For this review, use the dimensioned drawing (mm, ordinates from the lowest corner) and the shaded views. A direction names the side the tool comes from. Round coordinates to 2 decimals unless told otherwise and drop trailing zeros. Write each loop counter-clockwise with the first axis right and the second up, starting at its lowest first coordinate (ties: lowest second). Pieces come first, ordered by that corner, then holes. Notation, with made-up numbers: M -13.75,-15 L -2.75,-15 A13 ccw -2.75,-7 Z; hole C -20,66.5 d8. An arc over 180 degrees is marked long. Answer in a Markdown table with one row per item.
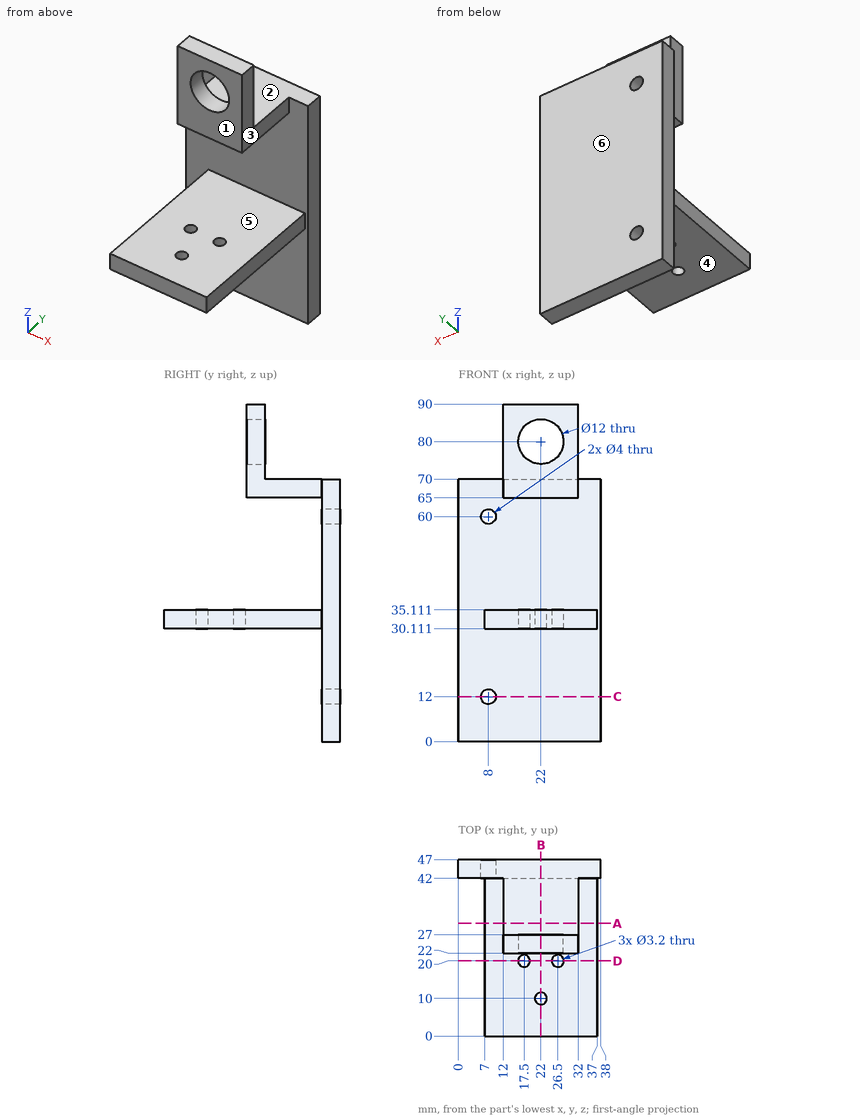
Q1. Take a section at A-A (y = 30). State the section outline as (x, z) points, then the cut area to 3 significant figures.
Found:
| item | result |
|---|---|
| outline | M 7,30.11 L 37,30.11 L 37,35.11 L 7,35.11 Z; M 12,65 L 32,65 L 32,70 L 12,70 Z |
| area | 250 mm² |
Q2. Machinability: for the marked faces 1, 2 and 3, which of the approach directions +Z, -Z, +X, -X, +Y, -Y give a long, thin tool a straight path to every point of the face, cutting with its end or side? Answer none if there is none.
Found:
| item | result |
|---|---|
| face 1 | +Z, +X, -X, -Y |
| face 2 | +Z, +X, -X, +Y |
| face 3 | +Z, +X, -Y |
Q3. For probe 1 along Z at (x, y) = (21.5, 22.5); probe 2 along Z at (x, y) = (26, 34.5); probe 3 along Y at (x, z) = (36.5, 56), list the stretches that pass through material, from the lowest coordinate up.
Found:
| item | result |
|---|---|
| probe 1 | 30.11 to 35.11, 65 to 74.02, 85.98 to 90 |
| probe 2 | 30.11 to 35.11, 65 to 70 |
| probe 3 | 42 to 47 |
Q4. Mouldability with a two-part tool opening along Z and no side actions: class the marked faces 4, 5 and 6 as +Z half, -Z half, draft (parallel to the pull), parting line (faces both ways), or undercut.
Found:
| item | result |
|---|---|
| face 4 | -Z half |
| face 5 | undercut |
| face 6 | draft |
Q5. Insertion check: P1, Ø10, axis at x = 10, y = 38, coming from the +Z side; P2, Ø12, axis at x = 15.5, y = 35, coming from the -Z side; P3, Ø14, axis at x = 22, z = 80, coming from the +Y side. Each pin has a flat end and moves straight along its axis. Give the tip position at first contact, or say it passes through.
Found:
| item | result |
|---|---|
| P1 | z = 70 |
| P2 | z = 30.11 |
| P3 | y = 27 |
Q6. Take a section at D-D (y = 20). State the section outline as (x, z) points.
Found:
| item | result |
|---|---|
| outline | M 7,30.11 L 15.9,30.11 L 15.9,35.11 L 7,35.11 Z; M 19.1,30.11 L 24.9,30.11 L 24.9,35.11 L 19.1,35.11 Z; M 28.1,30.11 L 37,30.11 L 37,35.11 L 28.1,35.11 Z |
Q7. Take a section at B-B (x = 22). State the section outline as (y, z) points, then the cut area to 3 significant figures.
Found:
| item | result |
|---|---|
| outline | M 0,30.11 L 8.4,30.11 L 8.4,35.11 L 0,35.11 Z; M 11.6,30.11 L 42,30.11 L 42,0 L 47,0 L 47,70 L 27,70 L 27,74 L 22,74 L 22,65 L 42,65 L 42,35.11 L 11.6,35.11 Z; M 22,86 L 27,86 L 27,90 L 22,90 Z |
| area | 684 mm² |
Q8. Take a section at C-C (z = 12). State the section outline as (x, y) points, then the cut area to 3 significant figures.
Found:
| item | result |
|---|---|
| outline | M 0,42 L 6,42 L 6,47 L 0,47 Z; M 10,42 L 38,42 L 38,47 L 10,47 Z |
| area | 170 mm² |
